from build123d import *

# Parameters (mm, degrees)
SKETCH1_R           = 30
BOSS_EXTRUDE1_DEPTH = 175
SKETCH3_W           = 10
SKETCH3_H           = 35


with BuildPart() as part:
    # Sketch1 → Boss-Extrude1 (new body)
    with BuildSketch(Plane(origin=(0, 0, 0), x_dir=(0, 0, -1), z_dir=(1, 0, 0))):
        Circle(SKETCH1_R)
    boss_extrude1 = extrude(amount=BOSS_EXTRUDE1_DEPTH)

    # Sketch3 → Revolve1 (revolve)
    with BuildSketch(Plane.XY, mode=Mode.PRIVATE) as revolve1_sk:
        with Locations((25, 17.5)):
            Rectangle(SKETCH3_W, SKETCH3_H)
        with BuildLine():
            Line((0, 0), (-45.458392513, 0))
            add(Edge.make_bspline(
                [(-45.458392513, 0), (-45.458392513, 20.183781855), (-30.991238831, 45), (0, 45)],
                knots=[0, 0, 0, 0, 1, 1, 1, 1], degree=3))
            Line((0, 45), (0, 0))
        make_face()
    revolve1 = revolve(revolve1_sk.sketch.rotate(Axis((-100.078673334, 0, 0), (1, 0, 0)), 90), axis=Axis((-100.078673334, 0, 0), (1, 0, 0)))

    # Mirror1: Boss-Extrude1, Revolve1 across plane
    add(boss_extrude1.mirror(Plane(origin=(175, 0, 0), x_dir=(0, 0, 1), z_dir=(1, 0, 0))))
    add(revolve1.mirror(Plane(origin=(175, 0, 0), x_dir=(0, 0, 1), z_dir=(1, 0, 0))))


solid = part.part
Can you work these out from the model? Positions are in its coordinate system, mm. Give positions to 0.01 mm unless a question says otherwise; leave off trailing zeros. Loops run counter-clockwise (first coordinate to the right, second up) from the corner with the lowest first, then second, coordinate; pieces in that order, holes last. Notation, with made-up numbers: (7, 28) - (17, 28) arc R21 cw to (17, 58) - close; hole circle Ø8 at (25, 76). An arc over 180 degrees is marked (long way). Return JSON: item names as keys, results as strings.
1. If I drill on line 1 (X direction, y = -31, z = -0.5); line 2 (X direction, y = 6, z = -30); line 3 (X direction, y = -0.5, z = 38), over which ranges is the centre line in solid material (lowest first)?
Output values:
{"line 1": "x = -33.52 to 0, 20 to 30, 320 to 330, 350 to 383.52", "line 2": "x = -33.89 to 0, 20 to 30, 320 to 330, 350 to 383.89", "line 3": "x = -25.28 to 0, 350 to 375.28"}
2. I'm going to push flat-ended pins straight in: pin 1 Ø4 at (y, z) = (-22.5, -15) entering from -X; pin 2 Ø10 at (x, z) = (212.5, -29.5) entering from -Y; pin 3 Ø2 at (x, z) = (246.5, -24.5) entering from -Y. Where does each tip first touch, or does it pass through?
Output values:
{"pin 1": "stops at x = -38.08", "pin 2": "stops at y = -17.31", "pin 3": "stops at y = -18.65"}
3. I want a section at A-A on x = 66. Please give me the cut outline in (y, z).
Output values:
{"outline": "circle Ø60 at (0, 0)"}
